```python
from build123d import *

# Parameters (mm, degrees)
F0_W     = 50.8
F0_H     = 50.8
F1_DEPTH = 876.3
F2_W     = 44.45
F2_H     = 44.45
F3_DEPTH = 876.3
F4_R     = 9.525


with BuildPart() as f1:
    # F0 (on Right) → F1 (new body)
    with BuildSketch(Plane.YZ):
        with Locations((25.4, 25.4)):
            Rectangle(F0_W, F0_H)
    extrude(amount=-F1_DEPTH)

    # F2 (on face) → F3 (cut)
    with BuildSketch(Plane.YZ):
        with Locations((25.4, 25.4)):
            Rectangle(F2_W, F2_H)
    extrude(amount=-F3_DEPTH, mode=Mode.SUBTRACT)

    # F4
    f4_edges = [f1.edges().sort_by_distance(p)[0] for p in [
        (-438.15, 3.175, 3.175),
        (-438.15, 47.625, 3.175),
        (-438.15, 47.625, 47.625),
        (-438.15, 3.175, 47.625),
        (-438.15, 50.8, 0),
        (-438.15, 50.8, 50.8),
        (-438.15, 0, 50.8),
        (-438.15, 0, 0),
    ]]
    fillet(f4_edges, radius=F4_R)


solid = f1.part
```
Work out the finished part from the listing and answer in its coordinate system (mm). A direction names the side the tool comes from. Round coordinates to 2 decimals unless told otherwise and drop trailing zeros. Write each loop counter-clockwise with the first axis right and the second up, starting at its lowest first coordinate (ties: lowest second). Pieces come first, ordered by that corner, then holes. Notation, with made-up numbers: (8, -2) - (61, -2) arc R24 cw to (61, 21) - close; hole circle Ø7 at (-15.75, -28.5). An arc over 180 degrees is marked (long way). Return JSON: item names as keys, results as strings. Group by question number.
Q1. The mould has two halves that part along Z. Classify faces 3 (the flat face through (-432, 3.175, 25)), 4 (the flat face through (-432, 25, 3.175)), 5 (the flat face through (-432, 25, 0)), 6 (the flat face through (-876.3, 27, 3)): released by +Z, released by -Z, zero draft, split by the parting line, or undercut.
Q2. The part is cut by section B-B on x = -683.5. Write down the section's boundary in (y, z) (3 decimals), then the cut area to 3 significant figures.
Q3. The part is cut by section A-A on y = 29.5. Write down the section's boundary in (x, z) (3 decimals), then the cut area to 3 significant figures.
Q4. For faces 1 (the flat face through (-432, 0, 25)), 2 (the flat face through (-432, 25, 47.625)), determine the directions among +Z, -Z, +X, -X, +Y, -Y from which every point of the face is accessible in a straight line to the end or side of a thin tool.
Q5. Find the intervals of material crossed by L1, parallel to Y at x = -813, z = 32 (3 decimals); L2, parallel to Z at x = -620.5, y = 7, in increasing order.
Q6. This flat-tipped pin is pushed along its axis until it touches: pin 1 Ø2 at (y, z) = (43.5, 43) entering from +X. Where does it stop, or does it pass through?
Solved:
{
 "1": {"face 3": "undercut", "face 4": "undercut", "face 5": "released by -Z", "face 6": "zero draft"},
 "2": {"outline": "(0, 9.525) arc R9.525 ccw to (9.525, 0) - (41.275, 0) arc R9.525 ccw to (50.8, 9.525) - (50.8, 41.275) arc R9.525 ccw to (41.275, 50.8) - (9.525, 50.8) arc R9.525 ccw to (0, 41.275) - close; hole (3.175, 12.7) arc R9.525 ccw to (12.7, 3.175) - (38.1, 3.175) arc R9.525 ccw to (47.625, 12.7) - (47.625, 38.1) arc R9.525 ccw to (38.1, 47.625) - (12.7, 47.625) arc R9.525 ccw to (3.175, 38.1) - close", "area": "605 mm²"},
 "3": {"outline": "(-876.3, 0) - (0, 0) - (0, 3.175) - (-876.3, 3.175) - close; (-876.3, 47.625) - (0, 47.625) - (0, 50.8) - (-876.3, 50.8) - close", "area": "5,560 mm²"},
 "4": {"face 1": "+Z, -Z, +X, -X, -Y", "face 2": "+X, -X"},
 "5": {"L1": "0 to 3.175, 47.625 to 50.8", "L2": "0.34 to 5.07, 45.73 to 50.46"},
 "6": {"pin 1": "through"}
}
